Check sheet for the drawn part. Datum: minimum x, y, z corner. Units: mm. A direction names the side the tool comes from. Round coordinates to 2 decimals unless told otherwise and drop trailing zeros. Write each loop counter-clockwise with the first axis right and the second up, starting at its lowest first coordinate (ties: lowest second). Pieces come first, ordered by that corner, then holes. Notation, with made-up numbers: (-36.75, -19) - (-11.75, -19) arc R28 cw to (-11.75, 15) - close; hole circle Ø4 at (-20, -13). An arc over 180 degrees is marked (long way). Write each question's results on one line, items separated by ' | '.
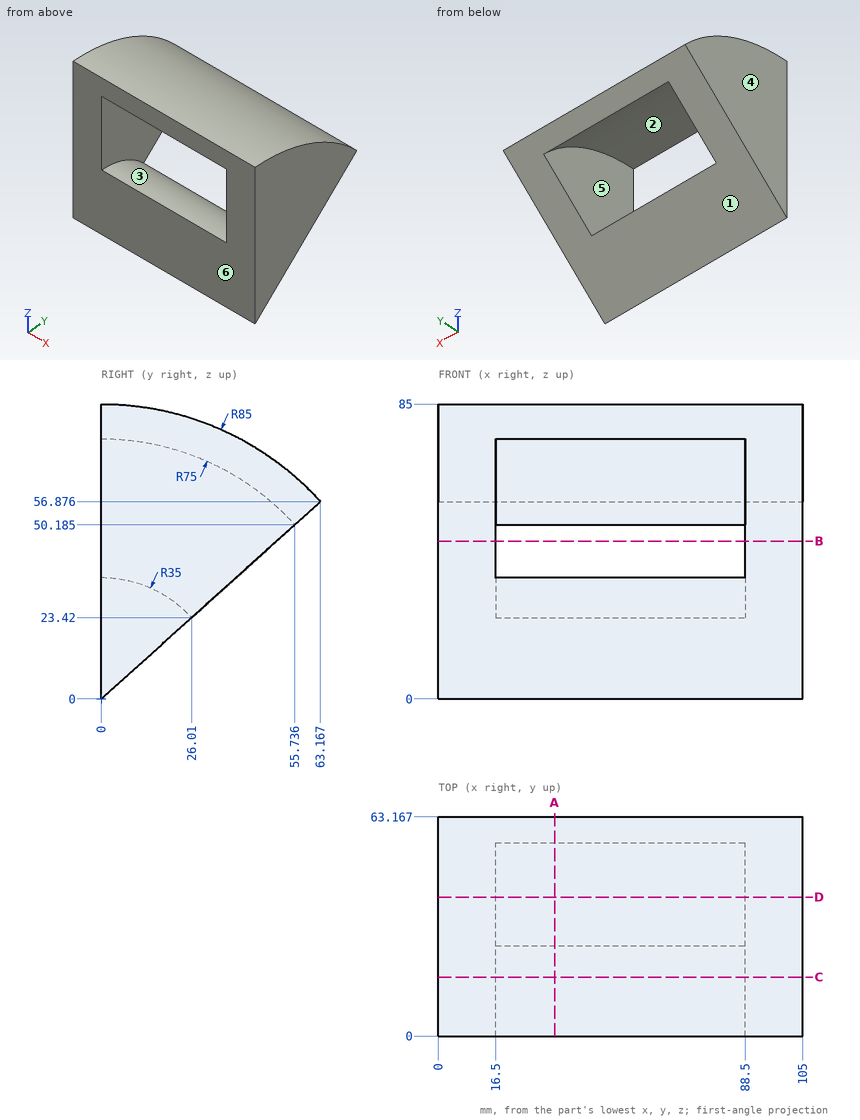
(1) Section check D-D (y = 40). Record the cut outline in (x, z).
Answer:
outline: (0, 36.02) - (16.5, 36.02) - (16.5, 63.44) - (88.5, 63.44) - (88.5, 36.02) - (105, 36.02) - (105, 75) - (0, 75) - close
(2) Section check A-A (x = 33.5). Record the cut outline in (y, z) (1 decimal).
Answer:
outline: (0, 0) - (26, 23.4) arc R35 ccw to (0, 35) - close; (0, 75) arc R75 cw to (55.7, 50.2) - (63.2, 56.9) arc R85 ccw to (0, 85) - close
(3) Go/stop test with flat-tipped pins: pin 1 Ø1.5 at (x, z) = (31.5, 28.5) entering from +Y; pin 2 Ø2 at (x, y) = (83.5, 44) entering from -Z; pin 3 Ø6 at (x, y) = (85, 46.5) entering from -Z (1 decimal). Record where each tip stops, or that it passes through.
Answer:
pin 1: y = 21.33 | pin 2: z = 60 | pin 3: z = 56.3
(4) Thickness scan on L1, parallel to X at y = 29.5, z = 55.5; L2, parallel to Z at x = 80, y = 39 (1 decimal); L3, parallel to Y at x = 74.5, z = 58.5 (1 decimal). Record the ranges inside material, lowest first.
Answer:
L1: 0 to 16.5, 88.5 to 105 | L2: 64.1 to 75.5 | L3: 46.9 to 61.7
(5) Set-up check for the marked faces 1, 2 and 3: record each of +Z, -Z, +X, -X, +Y, -Y from which the full face is reachable in a straight line by a thin tool's end or side.
Answer:
face 1: -Z, +X, -X, +Y | face 2: -Y | face 3: +Y
(6) Mould release check, pull along X, two halves, no side actions. Record for the marked faces 4, 5 and 6: released by +X, released by -X, zero draft, split by the parting line, or undercut.
Answer:
face 4: released by -X | face 5: undercut | face 6: zero draft
(7) Section check C-C (y = 17). Record the cut outline in (x, z), plus the area to 3 significant figures.
Answer:
outline: (0, 15.31) - (105, 15.31) - (105, 83.28) - (0, 83.28) - close; hole (16.5, 30.59) - (88.5, 30.59) - (88.5, 73.05) - (16.5, 73.05) - close | area: 4,080 mm2
(8) Section check B-B (z = 45.5). Record the cut outline in (x, y).
Answer:
outline: (0, 0) - (16.5, 0) - (16.5, 50.53) - (0, 50.53) - close; (88.5, 0) - (105, 0) - (105, 50.53) - (88.5, 50.53) - close
